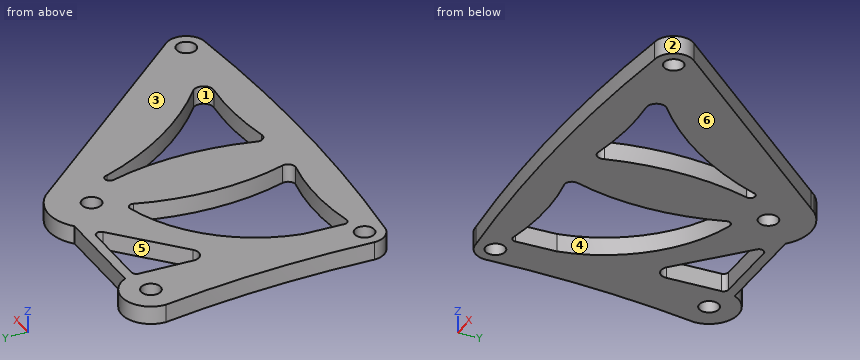
Autodesk Inventor part; units mm, degrees
ref_plane "YZ Plane" through (0, 0, 0) normal (1, 0, 0) x (0, 1, 0)
ref_plane "XZ Plane" through (0, 0, 0) normal (0, 1, 0) x (-1, 0, 0)
ref_plane "XY Plane" through (0, 0, 0) normal (0, 0, 1) x (1, 0, 0)
sketch "Sketch1" plane through (0, 0, 0) normal (0, 0, 1) x (1, 0, 0)
  line L0 (-110, 70) -> (110, 70) construction
  line L1 (110, 70) -> (110, -70) construction
  line L2 (110, -70) -> (-110, -70) construction
  line L3 (-110, -70) -> (-110, 70) construction
  circle A0 centre (-90.0138, 55) radius 5
  circle A1 centre (-90.0214, -55) radius 5
  circle A2 centre (89.9786, -55) radius 5
  circle A3 centre (-10.4773, 45) radius 5
  line L4 (-67, 0) -> (-42, 0) construction
  line L5 (-42, 0) -> (-42, -30) construction
  line L6 (-42, -30) -> (-67, -30) construction
  line L7 (-67, -30) -> (-67, 0) construction
  circle A4 centre (-54.5, -19) radius 10 construction
  arc A5 (-76.3936, 61.2841) -> (-104.4102, 50.7876) centre (-90.0138, 55) ccw
  arc A6 (-99.9609, -53.9017) -> (-88.1312, -64.8197) centre (-90.0214, -55) ccw
  arc A7 (-100.0214, -55.005) -> (-105.0138, 54.9917) centre (-644.4166, -24.602) ccw
  line L8 (-35.5883, 51.8649) -> (-68.1439, 22.1865)
  line L9 (-75.3098, 53.8204) -> (-76.5077, 26.0974)
  line L10 (-78.8288, -29.0174) -> (-79.7785, -49.89)
  arc A8 (89.9786, -65) -> (97.6038, -48.5303) centre (89.9786, -55) ccw
  line L11 (4.9567, 60.6642) -> (97.6038, -48.5303)
  arc A9 (4.9567, 60.6642) -> (-25.2559, 61.2841) centre (-10.4773, 45) ccw
  arc A10 (-76.5077, 26.0974) -> (-68.1439, 22.1865) centre (-71.5124, 25.8816) ccw
  line L12 (-76.3936, 61.2841) -> (-25.2559, 61.2841)
  line L13 (-72.8121, 56.2124) -> (-37.2725, 56.2124)
  arc A11 (-72.8121, 56.2124) -> (-75.3098, 53.8204) centre (-72.8121, 53.7124) ccw
  arc A12 (-35.5883, 51.8649) -> (-37.2725, 56.2124) centre (-37.2725, 53.7124) ccw
  arc A13 (-20.0641, 28.3268) -> (-21.4793, -47.6907) centre (99.5505, -11.922) ccw
  circle A14 centre (-63.5274, -9.3914) radius 3 construction
  circle A15 centre (-57.919, -6.3914) radius 3 construction
  circle A16 centre (-51.0643, -6.3914) radius 3 construction
  circle A17 centre (-45.5038, -9.3914) radius 3 construction
  arc A18 (-23.0905, 31.5363) -> (-78.8288, -29.0174) centre (-2.761, -43.1063) ccw
  arc A19 (-20.0641, 28.3268) -> (-23.0905, 31.5363) centre (-22.4335, 29.1241) ccw
  arc A20 (-25.0801, -52.5035) -> (-21.4793, -47.6907) centre (-25.0756, -48.7535) ccw
  arc A21 (-79.7785, -49.89) -> (-77.2605, -52.5035) centre (-77.2811, -50.0036) ccw
  arc A22 (-90.0214, -65) -> (89.9786, -65) centre (-0.0214, 742.5) ccw
  arc A23 (-25.0801, -52.5035) -> (-77.2605, -52.5035) centre (-51.1703, -178.0833) ccw
  arc A24 (89.9786, -65) -> (97.6038, -48.5303) centre (89.9786, -55) ccw
  arc A25 (51.3169, -49.4442) -> (6.7008, -51.3162) centre (35.2009, -197.9611) ccw
  arc A26 (7.4915, 57.6767) -> (-25.2559, 61.2841) centre (-10.4773, 45) ccw
  arc A27 (2.5412, -46.1517) -> (6.7008, -51.3162) centre (5.9854, -47.6351) ccw
  arc A28 (51.3169, -49.4442) -> (55.6269, -41.1897) centre (51.8562, -44.4734) ccw
  arc A29 (2.5412, -46.1517) -> (2.5412, 27.2773) centre (-130.6751, -9.4372) ccw
  arc A30 (7.4934, 27.7888) -> (2.5825, 27.1273) centre (4.9934, 27.7888) ccw
  arc A31 (7.4934, 27.7888) -> (55.6269, -41.1897) centre (157.8186, 81.4032) ccw
  point P0 (0, 0)
  point P1 (-90.7944, -64.9701)
  point P2 (-90.0214, -65)
  dimension "d1" = 70
  dimension "d2" = 70
  dimension "d5" = 10
  dimension "d6" = 10
  dimension "d7" = 10
  dimension "d8" = 10
  dimension "d9" = 55
  dimension "d10" = 55
  dimension "d11" = 55
  dimension "d12" = 180
  dimension "d16" = 45
  dimension "d17" = 42
  dimension "d18" = 30
  dimension "d19" = 0
  dimension "d20" = 25
  dimension "d21" = 20
  dimension "d25" = 19
  dimension "d26" = 12.5
  dimension "d68" = 30
  dimension "d70" = 20
  dimension "d71" = 20
  dimension "d74" = 10
  dimension "d75" = 5
  dimension "d76" = 5
  dimension "d77" = 6
  dimension "d78" = 6
  dimension "d79" = 6
  dimension "d80" = 6
  dimension "d81" = 5
  dimension "d84" = 7.5
  dimension "d88" = 5
  dimension "d92" = 7.5
  dimension "d93" = 10
  dimension "d94" = 5
extrude "Extrusion9" add sketch "Sketch1" along normal blind 9.4 contours L12 A9 L11 A8 A22 A6 A7 A5
equation "\"d26\" = 0.5 * d20"
properties part number "Bracket Concept MK11"
Part model, mm, in its own coordinate system. Face numbers are marked on the shaded views. A direction names the side the tool comes from. Coordinates: 2 decimals unless noted, no trailing zeros. Loops run counter-clockwise (first coordinate to the right, second up) from the corner with the lowest first, then second, coordinate; pieces in that order, holes last. Notation, with made-up numbers: (-0.5, 45.25) - (58.5, 45.25) arc R17 ccw to (58.5, 64.25) - close; hole circle Ø6 at (39, 19.5). An arc over 180 degrees is marked (long way). Write item = value, one per line. Start each with the question number.
Item 1: Cut at B-B, the plane y = 45. Give the cut face in (x, z), and give its area (4 significant figures).
Item 2: Wall check: L1, parallel to Y at x = -53, z = 2.25; L2, parallel to X at y = 4.5, z = 6.5; L3, parallel to X at y = 51, z = 5.5. Give the ranges that are in metal, low to high. Write a range as from..to.
Item 3: Mould opens along X. For the marked faces 1, 2, 3 and 4 say: released by +X, released by -X, zero draft, split by the parting line, or undercut.
Item 4: Flat gauge pins, fed straight in: pin 1 Ø2 at (y, z) = (-24, 6.5) entering from +X; pin 2 Ø1 at (x, z) = (36.5, 1.5) entering from -Y; pin 3 Ø2 at (y, z) = (36, 6.5) entering from +X. Where does each tip first touch, or does it go through?
Item 5: Cut at C-C, the plane z = 5.25. State how many separate pieces and enclosed holes the cut face has, and give its area (3 significant figures).
Item 6: Cut at D-D, the plane x = -44. Give the cut face in (y, z).
Item 7: Cut at A-A, the plane x = 21.5. Give the cut face in (y, z), and give its area (3 significant figures).
Item 8: 3-axis set-ups, long thin cutter, end or side, ignore diameter. For the marked faces 5 and 6: which of +Z, -Z, +X, -X, +Y, -Y reach the whole face in a straight line?
The answers:
q1.outline = (-103.63, 0) - (-75.69, 0) - (-75.69, 9.4) - (-103.63, 9.4) - close; (-43.12, 0) - (-15.48, 0) - (-15.48, 9.4) - (-43.12, 9.4) - close; (-5.48, 0) - (18.25, 0) - (18.25, 9.4) - (-5.48, 9.4) - close
q1.area = 745.5 mm2
q2.L1 = -68.27..-49.83, 15.72..35.99, 56.21..61.28
q2.L2 = -99.95..-63.74, -25.58..6.8, 17.97..52.61
q2.L3 = -104.44..-93.01, -87.01..-75.43, -36.54..13.16
q3.face_1 = undercut
q3.face_2 = released by +X
q3.face_3 = zero draft
q3.face_4 = undercut
q4.pin_1 = 77.64
q4.pin_2 = -69.2
q4.pin_3 = 26.73
q5.separate_pieces = 1
q5.enclosed_holes = 7
q5.area = 14,300 mm2
q6.outline = (-68.81, 0) - (-50.02, 0) - (-50.02, 9.4) - (-68.81, 9.4) - close; (22.35, 0) - (44.2, 0) - (44.2, 9.4) - (22.35, 9.4) - close; (56.21, 0) - (61.28, 0) - (61.28, 9.4) - (56.21, 9.4) - close
q7.outline = (-69.71, 0) - (-49.2, 0) - (-49.2, 9.4) - (-69.71, 9.4) - close; (-1.6, 0) - (41.17, 0) - (41.17, 9.4) - (-1.6, 9.4) - close
q7.area = 595 mm2
q8.face_5 = +Z, -Z
q8.face_6 = -Z, +X, -X, +Y, -Y
